Autodesk Inventor part; units mm, degrees
ref_plane "gba_XY" through (8.6, 0, 0) normal (1, 0, 0) x (0, 0, -1)
ref_plane "gba_YZ" through (8.6, 0, 0) normal (0, 0, -1) x (0, 1, 0)
ref_plane "gba_ZX" through (8.6, 0, 0) normal (0, 1, 0) x (1, 0, 0)
sketch "Sketch_1" plane through (0, 0, 0) normal (0, 1, 0) x (-1, 0, 0)
  line L0 (-8.6, 0) -> (0, 0)
  line L1 (0, 0) -> (0, -7.5)
  line L2 (0, -7.5) -> (-8.3113, -7.5)
  line L3 (-8.3113, -7.5) -> (-8.6, -7)
  line L4 (-8.6, -7) -> (-8.6, 0)
  line L5 (-8.6, 0) -> (0, 0)
revolve "Revolution1" add sketch "Sketch_1" angle 360 about axis through (8.6, 0, 0) along (1, 0, 0)
sketch "Sketch_2" plane through (0, 0, 0) normal (0, 1, 0) x (-1, 0, 0)
  line L0 (-50, 0) -> (50, 0)
  line L1 (0, -6.75) -> (-0.433, -7)
  line L2 (-0.433, -7) -> (-3.85, -7)
  line L3 (-3.85, -7) -> (-3.85, -7.5)
  line L4 (-3.85, -7.5) -> (0, -7.5)
  line L5 (0, -7.5) -> (0, -6.75)
revolve "Revolution2" cut sketch "Sketch_2" angle 360 about axis through (50, 0, 0) along (1, 0, 0)
sketch "Sketch_3" plane through (0, 0, 0) normal (0, 1, 0) x (-1, 0, 0)
  line L0 (-50, 0) -> (50, 0)
  line L1 (-3.85, -7.5) -> (-3.85, -7.3)
  line L2 (-3.85, -7.3) -> (-4.05, -7.5)
  line L3 (-4.05, -7.5) -> (-3.85, -7.5)
revolve "Revolution3" cut sketch "Sketch_3" angle 360 about axis through (50, 0, 0) along (1, 0, 0)
sketch "Sketch4" plane through (8.6, 0, 0) normal (1, 0, 0) x (0, 0, -1)
  point P0 (0, 0)
hole "Hole1" at (8.6, 0, 0) direction (-1, 0, 0) diameter 10.6 depth 8.6
ref_plane "gba_XY" through (8.6, 0, 0) normal (1, 0, 0) x (0, 0, -1)
ref_plane "gba_YZ" through (8.6, 0, 0) normal (0, 0, -1) x (0, 1, 0)
ref_plane "gba_ZX" through (8.6, 0, 0) normal (0, 1, 0) x (1, 0, 0)
properties part number "SCHUNK-9951430 Zentrierhuelse PGN-plus"
Here's how the part is built. I have some questions about the finished solid (model axes, mm). Round coordinates to 2 decimals unless told otherwise and drop trailing zeros. Order: outer loops, then holes, each group sorted by start corner. A loop starts at its lowest first (then second) coordinate and runs counter-clockwise, first axis right, second up. Notation, with made-up numbers: M -8.75,71 L 17.25,71 A15 ccw 17.25,83 Z; hole C 79.5,1 d8. An arc over 180 degrees is marked long. Answer as CSV lines item,"result".
Item 1: Please list where these lines run through material, in increasing order: L1, parallel to Y at x = 2.5, z = 0; L2, parallel to Y at x = 5.25, z = 0; L3, parallel to Z at x = 4.5, y = 0.5. Write a range as [from, to].
From the geometry:
L1,"[-7, -5.3], [5.3, 7]"
L2,"[-7.5, -5.3], [5.3, 7.5]"
L3,"[-7.48, -5.28], [5.28, 7.48]"
Item 2: Imagine slicing it at C-C on x = 6.75. List the corners of the cut face in (y, z) for me.
From the geometry:
outline,"C 0,0 d15; hole C 0,0 d10.6"
Item 3: We'd pull the mould along Y, two halves only. Please class faces 1 (the flat face through (8.6, 5, -3)), 2 (the cylindrical face through (2.165, -2.681, -6.466)), 3 (the cylindrical face through (4.24, 2.03, -4.896)): +Y half, -Y half, draft (parallel to the pull), parting line (faces both ways), or undercut.
From the geometry:
face 1,"draft"
face 2,"parting line"
face 3,"undercut"
Item 4: Imagine slicing it at A-A on z = 0. List the corners of the cut face in (x, y) for me, and give its area (3 significant figures).
From the geometry:
outline,"M 0,-6.75 L 0.43,-7 L 3.85,-7 L 3.85,-7.3 L 4.05,-7.5 L 8.31,-7.5 L 8.6,-7 L 8.6,-5.3 L 0,-5.3 Z; M 0,5.3 L 8.6,5.3 L 8.6,7 L 8.31,7.5 L 4.05,7.5 L 3.85,7.3 L 3.85,7 L 0.43,7 L 0,6.75 Z"
area,"33.7 mm2"
Item 5: For pin 1 (5 mm diameter, centred on x = 4.5, y = -4, fed in from -Z); pin 2 (7.5 mm diameter, centred on y = 3, z = 2, fed in from -X); pin 3 (1.5 mm diameter, centred on x = 4.5, z = -6, fed in from +Y); pin 4 (4 mm diameter, centred on x = 1, y = 4, fed in from +Z), each with a flat end and sliding along its axis, tell me the tip position at first contact or that it passes through.
From the geometry:
pin 1,"z = -7.35"
pin 2,"x = 0"
pin 3,"y = 5.36"
pin 4,"z = 6.71"
Item 6: Imagine slicing it at D-D on x = 3.5. List the corners of the cut face in (y, z) for me.
From the geometry:
outline,"C 0,0 d14; hole C 0,0 d10.6"
